from build123d import *

# Parameters (mm, degrees)
F1_DEPTH = 17.4625
F2_R     = 2.032
F4_DEPTH = 25.4
F5_START = -5.588
F5_DEPTH = 19.812
F3_R     = 2.032
F6_DEPTH = 25.4
F7_START = -4.572
F7_DEPTH = 20.828
F8_R     = 2.032
F9_R     = 1.27


with BuildPart() as f1:
    # F0 (on Front) → F1 (new body, symmetric)
    with BuildSketch(Plane.XZ):
        Polygon((63.5, 0), (0, 0), (0, -50.8), (7.62, -50.8), (7.62, -22.86), (22.86, -7.62), (63.5, -7.62), align=None)
    extrude(amount=F1_DEPTH, both=True)

    # F2 (on face) → F4 (cut)
    with BuildSketch(Plane.XY):
        with Locations((17.78, 0)):
            Circle(F2_R)
        with Locations((50.8, 0)):
            Circle(F2_R)
    extrude(amount=-F4_DEPTH, mode=Mode.SUBTRACT)

    # F2 (on face) → F5 (cut)
    with BuildSketch(Plane.XY.offset(F5_START)):
        Polygon((21.844, 2.346351494), (17.78, 4.692702988), (13.716, 2.346351494), (13.716, -2.346351494), (17.78, -4.692702988), (21.844, -2.346351494), align=None)
        with Locations((17.78, 0)):
            Circle(F2_R, mode=Mode.SUBTRACT)
        Polygon((54.864, 2.346351494), (50.8, 4.692702988), (46.736, 2.346351494), (46.736, -2.346351494), (50.8, -4.692702988), (54.864, -2.346351494), align=None)
        with Locations((50.8, 0)):
            Circle(F2_R, mode=Mode.SUBTRACT)
    extrude(amount=-F5_DEPTH, mode=Mode.SUBTRACT)

    # F3 (on face) → F6 (cut)
    with BuildSketch(Plane(origin=(0, 0, 0), x_dir=(0, -1, 0), z_dir=(-1, 0, 0))):
        with Locations((0, -25.4)):
            Circle(F3_R)
    extrude(amount=-F6_DEPTH, mode=Mode.SUBTRACT)

    # F3 (on face) → F7 (cut)
    with BuildSketch(Plane(origin=(0, 0, 0), x_dir=(0, -1, 0), z_dir=(-1, 0, 0)).offset(F7_START)):
        Polygon((-2.346351494, -29.464), (2.346351494, -29.464), (4.692702988, -25.4), (2.346351494, -21.336), (-2.346351494, -21.336), (-4.692702988, -25.4), align=None)
        with Locations((0, -25.4)):
            Circle(F3_R, mode=Mode.SUBTRACT)
    extrude(amount=-F7_DEPTH, mode=Mode.SUBTRACT)

    # F8
    f8_edges = [f1.edges().sort_by_distance(p)[0] for p in [
        (63.5, 0, -7.62),
        (7.62, 0, -50.8),
        (7.62, -10.344367, -22.86),
        (7.62, 10.344367, -22.86),
        (22.86, 0, -7.62),
        (0, 0, 0),
    ]]
    fillet(f8_edges, radius=F8_R)

    # F9
    f9_edges = [f1.edges().sort_by_distance(p)[0] for p in [
        (32.766, -17.4625, 0),
        (32.766, 17.4625, 0),
    ]]
    fillet(f9_edges, radius=F9_R)


solid = f1.part
Design review of the part built by this model. Coordinates are the model's own, in mm. A direction names the side the tool comes from. Coordinates: 2 decimals unless noted, no trailing zeros. Order: outer loops, then holes, each group sorted by start corner. A loop starts at its lowest first (then second) coordinate and runs counter-clockwise, first axis right, second up.
Item 1: For pin 1 Ø4 at (y, z) = (2, -25) entering from +X; pin 2 Ø10.5 at (x, y) = (48.5, 5.5) entering from -Z; pin 3 Ø5 at (y, z) = (0, -9.5) entering from +X, all flat-tipped, find the tip position at first contact; note any pin that passes through.
Item 2: Take a section at D-D, the plane x = 54. Write out the cut boundary in (y, z).
Item 3: Take a section at A-A, the plane y = 0. Count the separate pieces of the cut face and the enclosed holes in it, then the cut area to 3 significant figures.
Item 4: For line 1 (Y direction, x = 17.78, z = -3.55); line 2 (X direction, y = 0, z = -45); line 3 (Z direction, x = 44, y = 5), list the stretches that pass through material, from the lowest coordinate up.
Item 5: Take a section at B-B, the plane z = -20. Write out the cut boundary in (x, y), then the cut area to 3 significant figures.
Item 6: The part is to be moulded in two halves that separate along Y. For faces 4 (the flat face through (52.86, 3.503, -6.59)), 5 (the flat face through (18, 17.462, -11)), 6 (the flat face through (13.58, -0.24, -16.9)), say which applies: pulls with the +Y half, pulls with the -Y half, needs draft (parallel to the pull), parting line crosses it, or undercut.
Item 7: Take a section at C-C, the plane y = -7. Write out the cut boundary in (x, z).
Item 8: For faces 1 (the flat face through (42, 0, -7.62)), 2 (the cylindrical face through (2.254, 0.44, -27.384)), 3 (the flat face through (13.716, 0, -11)), list the 3-axis set-ups (+Z, -Z, +X, -X, +Y, -Y) from which the entire face can be reached by the end or side of a thin tool; tool diameter is ignored.
The answers:
1. pin 1: stops at x = 4.57
1. pin 2: stops at z = -7.62
1. pin 3: stops at x = 62.93
2. outline: (-17.46, -7.62) - (-2.85, -7.62) - (-2.85, -5.59) - (2.85, -5.59) - (2.85, -7.62) - (17.46, -7.62) - (17.46, -1.27) arc R1.27 ccw to (16.19, 0) - (-16.19, 0) arc R1.27 ccw to (-17.46, -1.27) - close
3. separate pieces: 4
3. enclosed holes: 0
3. area: 762 mm2
4. line 1: y = -17.46 to -2.03, 2.03 to 17.46
4. line 2: x = 0 to 7.62
4. line 3: z = -7.62 to 0
5. outline: (0, -16.19) arc R1.27 ccw to (1.27, -17.46) - (10.48, -17.46) - (10.48, 17.46) - (1.27, 17.46) arc R1.27 ccw to (0, 16.19) - close
5. area: 365 mm2
6. face 4: undercut
6. face 5: pulls with the +Y half
6. face 6: needs draft
7. outline: (0, -50.8) - (5.59, -50.8) arc R2.03 ccw to (7.62, -48.77) - (7.62, -23.7) arc R2.03 cw to (8.22, -22.26) - (22.26, -8.22) arc R2.03 cw to (23.7, -7.62) - (61.47, -7.62) arc R2.03 ccw to (63.5, -5.59) - (63.5, 0) - (2.03, 0) arc R2.03 ccw to (0, -2.03) - close
8. face 1: -Z, +X, +Y, -Y
8. face 2: +X, -X
8. face 3: -Z
